Design review of the part built by this model. Coordinates are the model's own, in mm. Face numbers are marked on the shaded views. A direction names the side the tool comes from. Coordinates: 2 decimals unless noted, no trailing zeros. Loops run counter-clockwise (first coordinate to the right, second up) from the corner with the lowest first, then second, coordinate; pieces in that order, holes last. Notation, with made-up numbers: M -6.75,44 L 52.25,44 A25 ccw 52.25,56 Z; hole C 2.25,-25 d8. An arc over 180 degrees is marked long. Put each result on its own line as item: value. Start each with the question number.
(1) For probe 1 along X at (y, z) = (-2, 86); probe 2 along X at (y, z) = (-3, 38.1); probe 3 along X at (y, z) = (-6, 38.1), list the stretches that pass through material, from the lowest coordinate up. Write a range as [from, to].
(2) The part is to be moulded in two halves that separate along Y. For the marked faces 3, 4 and 5, say which applies: +Y half, -Y half, draft (parallel to the pull), parting line (faces both ways), or undercut.
(3) For the marked faces 1 and 2, list the 3-axis set-ups (+Z, -Z, +X, -X, +Y, -Y) from which the entire face can be reached by the end or side of a thin tool; tool diameter is ignored.
(4) Clearance check with flat-ended pins moving along their axes: pin 1 (23 mm diameter, centred on x = 59.14, z = 38.1, fed in from +Y); pin 2 (10 mm diameter, centred on y = -5.5, z = 24.5, fed in from +X); pin 3 (10 mm diameter, centred on y = 2, z = 114, fed in from -X); pin 4 (1.5 mm diameter, centred on x = 27.5, y = 7, fed in from +Z). State where each tip first meets the part, or that it passes through.
(5) Take a section at B-B, the plane z = 48. Count the separate pieces of the cut face and the enclosed holes in it, then the cut area to 3 significant figures.
(6) Take a section at A-A, the plane y = 6.25. Give the boundary of the cut face in (x, z) (1 decimal), then the cut area to 3 significant figures.
```python
from build123d import *

# Parameters (mm, degrees)
F1_DEPTH = 9.525
F2_R     = 5.08


# Not quite as in the source:
# - a feature names something its author has since deleted; it is built from what else it names


with BuildPart() as f1:
    # F0 (on Front) → F1 (new body, symmetric)
    with BuildSketch(Plane.XZ):
        with BuildLine():
            Line((0, 15.875), (0, 0))
            ThreePointArc((0, 0), (13.2614611296, 0.8692020844), (26.2960149824, 3.461936049))
            Line((26.2960149824, 3.461936049), (108.6220112368, 25.5211202615))
            ThreePointArc((108.6220112368, 25.5211202615), (149.3535245302, 52.7370473342), (165.1, 99.1246682247))
            Line((165.1, 99.1246682247), (165.1, 117.475))
            Line((165.1, 117.475), (63.5, 117.475))
            Line((63.5, 117.475), (63.5, 106.8842132454))
            ThreePointArc((63.5, 106.8842132454), (45.4987113259, 57.6973247485), (0, 31.75))
            Line((0, 31.75), (0, 15.875))
        make_face()
        with BuildLine():
            ThreePointArc((71.8357677815, 38.1), (47.023562507, 34.2810363463), (69.5389987439, 45.3844207417))
            ThreePointArc((69.5389987439, 45.3844207417), (71.247973056, 41.9189636537), (71.8357677815, 38.1))
        make_face(mode=Mode.SUBTRACT)
        with BuildLine():
            ThreePointArc((117.6539419454, 79.0748666718), (120.8582687804, 72.5771346319), (121.9603838907, 65.4165777812))
            ThreePointArc((121.9603838907, 65.4165777812), (105.3084407414, 42.7061928915), (78.6418258361, 51.7582888906))
            ThreePointArc((78.6418258361, 51.7582888906), (84.4895950001, 84.9226358359), (117.6539419454, 79.0748666718))
        make_face(mode=Mode.SUBTRACT)
        with BuildLine():
            ThreePointArc((149.86, 92.7331555624), (140.9789636537, 80.6209502879), (126.7567690375, 85.4487348208))
            ThreePointArc((126.7567690375, 85.4487348208), (133.3410363463, 104.8453608369), (149.86, 92.7331555624))
        make_face(mode=Mode.SUBTRACT)
    extrude(amount=F1_DEPTH, both=True)

    # F2
    f2_edges = [f1.edges().sort_by_distance(p)[0] for p in [
        (45.498711, -9.525, 57.697325),
        (63.5, -9.525, 112.179607),
        (63.5, 9.525, 112.179607),
        (165.1, -9.525, 108.299834),
        (149.353525, -9.525, 52.737047),
        (13.261461, 9.525, 0.869202),
    ]]
    fillet(f2_edges, radius=F2_R)


solid = f1.part
```
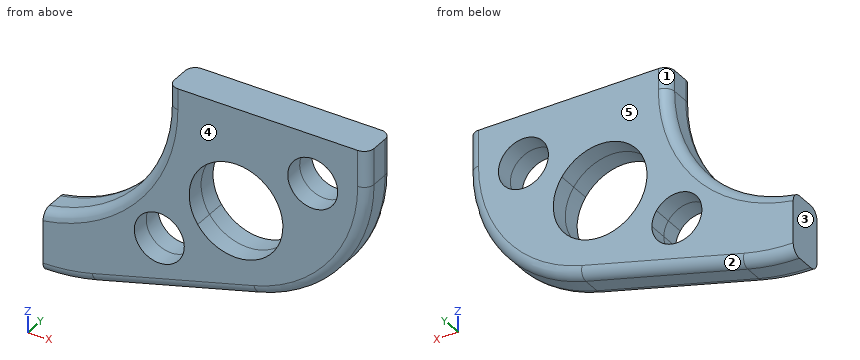
Computed values:
1. probe 1: x = [60.58, 86.17], [110.12, 126.39], [147.93, 163.96]
1. probe 2: x = [20.09, 46.44], [71.84, 134.53]
1. probe 3: x = [20.65, 46.44], [71.84, 134.13]
2. face 3: draft
2. face 4: -Y half
2. face 5: +Y half
3. face 1: +Z, -X, +Y
3. face 2: -Z, +X, +Y
4. pin 1: passes through
4. pin 2: stops at x = 119.73
4. pin 3: stops at x = 63.5
4. pin 4: stops at z = 41.99
5. separate pieces: 3
5. enclosed holes: 0
5. area: 1,140 mm^2
6. outline: M 0,0.3 A101.3 ccw 26.2,3.8 L 108.5,25.8 A75.9 ccw 164.8,99.1 L 164.8,117.5 L 63.8,117.5 L 63.8,106.9 A76.5 cw 0,31.4 Z; hole C 59.1,38.1 d25.4; hole C 98.1,65.4 d47.6; hole C 137.2,92.7 d25.4
6. area: 8,470 mm^2
